from build123d import *

# Parameters (mm, degrees)
SKETCH1_W           = 25
SKETCH1_H           = 34
BOSS_EXTRUDE1_DEPTH = 5
SKETCH2_W           = 10
SKETCH2_H           = 34
BOSS_EXTRUDE2_DEPTH = 51
SKETCH3_R           = 2.8
CUT_EXTRUDE1_DEPTH  = 41
CHAMFER1_SIZE       = 4
FILLET1_R           = 4
FILLET2_R           = 4
SKETCH4_R           = 0.85
CUT_EXTRUDE2_DEPTH  = 41
SKETCH5_W           = 10
SKETCH5_H           = 20
BOSS_EXTRUDE3_DEPTH = 6
CHAMFER3_SIZE       = 15
FILLET4_R           = 10
SKETCH7_R           = 0.9
SKETCH7_R_2         = 0.85
CUT_EXTRUDE3_DEPTH  = 13


with BuildPart() as part:
    # Sketch1 → Boss-Extrude1 (new body)
    with BuildSketch(Plane(origin=(0, 0, 0), x_dir=(1, 0, 0), z_dir=(0, 1, 0))):
        Rectangle(SKETCH1_W, SKETCH1_H)
    extrude(amount=BOSS_EXTRUDE1_DEPTH)

    # Sketch2 → Boss-Extrude2 (add)
    with BuildSketch(Plane(origin=(0, 5, 0), x_dir=(1, 0, 0), z_dir=(0, 1, 0))):
        Rectangle(SKETCH2_W, SKETCH2_H)
    extrude(amount=BOSS_EXTRUDE2_DEPTH)

    # Sketch3 → Cut-Extrude1 (cut)
    with BuildSketch(Plane.ZY.offset(5)):
        with Locations((0, 46)):
            Circle(SKETCH3_R)
    extrude(amount=-CUT_EXTRUDE1_DEPTH, mode=Mode.SUBTRACT)

    # Chamfer1
    chamfer1_edges = [part.edges().sort_by_distance(p)[0] for p in [
        (-12.5, 5, 0),
        (12.5, 5, 0),
    ]]
    chamfer(chamfer1_edges, length=CHAMFER1_SIZE)

    # Fillet1
    # the kernel refuses this fillet: 4 mm, written as the material it adds along each edge
    with BuildSketch(Plane(origin=(5, 5, 17), x_dir=(1, 0, 0), z_dir=(0, 0, -1)), Plane(origin=(-5, 5, -17), x_dir=(-1, 0, 0), z_dir=(0, 0, 1))) as fillet1_piece_1:
        with BuildLine():
            CenterArc((4, -3.968626967), FILLET1_R, 97.180755781, 82.819244219)
            Line((0, -3.968626967), (-0.08, -3.968626967))
            Line((-0.08, -3.968626967), (-0.08, 0))
            Line((-0.08, 0), (0, 0.08))
            ThreePointArc((0, 0.08), (1.75, 0.08), (3.49, 0.079372539))
            Line((3.49, 0.079372539), (3.5, 0))
        make_face()
    extrude(amount=34)

    # Fillet2
    fillet2_edges = [part.edges().sort_by_distance(p)[0] for p in [
        (8.5, 5, 0),
        (-8.5, 5, 0),
    ]]
    fillet(fillet2_edges, radius=FILLET2_R)

    # Sketch4 → Cut-Extrude2 (cut)
    with BuildSketch(Plane.ZY.offset(5)):
        with Locations((6, 29.968626967)):
            Circle(SKETCH4_R)
        with Locations((13, 29.968626967)):
            Circle(SKETCH4_R)
        with Locations((2.5, 29.968626967)):
            Circle(SKETCH4_R)
        with Locations((9.5, 29.968626967)):
            Circle(SKETCH4_R)
    extrude(amount=-CUT_EXTRUDE2_DEPTH, mode=Mode.SUBTRACT)

    # Sketch5 → Boss-Extrude3 (add)
    with BuildSketch(Plane(origin=(0, 0, -17), x_dir=(-1, 0, 0), z_dir=(0, 0, -1))):
        with Locations((0, 46)):
            Rectangle(SKETCH5_W, SKETCH5_H)
    extrude(amount=BOSS_EXTRUDE3_DEPTH)

    # Chamfer3
    # the kernel refuses this chamfer: 15 mm, written as the material it adds along each edge
    with BuildSketch(Plane(origin=(-5, 36, -17), x_dir=(0, -0.9996219169112968, 0.02749587661058632), z_dir=(1, 0, 0))) as chamfer3_piece_1_section:
        Polygon((CHAMFER3_SIZE * 0.999621916911, CHAMFER3_SIZE * 0.0274958766106), (-CHAMFER3_SIZE * 0.0274958766106, CHAMFER3_SIZE * 0.999621916911), (0, 0), align=None)
    chamfer3_piece_1 = extrude(amount=10, mode=Mode.PRIVATE)
    chamfer3_piece_1 = split(chamfer3_piece_1, bisect_by=Plane(origin=(0, 29.791642651, -23), z_dir=(0, 0, 1)), keep=Keep.TOP, mode=Mode.PRIVATE)
    add(chamfer3_piece_1)

    # Fillet4
    fillet4_edges = [part.edges().sort_by_distance(p)[0] for p in [
        (0, 56, 17),
        (0, 56, -23),
    ]]
    fillet(fillet4_edges, radius=FILLET4_R)

    # Sketch7 → Cut-Extrude3 (cut)
    with BuildSketch(Plane(origin=(5, 0, 0), x_dir=(0, 0, -1), z_dir=(1, 0, 0))):
        with Locations((13.030614343, 27.851199121)):
            Circle(SKETCH7_R)
        with Locations((19.374768852, 30.809526953)):
            Circle(SKETCH7_R_2)
    extrude(amount=-CUT_EXTRUDE3_DEPTH, mode=Mode.SUBTRACT)


solid = part.part
Could you check a few things on this model? Use its own coordinates, in mm. A direction names the side the tool comes from. Give positions to 0.01 mm unless a question says otherwise; leave off trailing zeros. Order: outer loops, then holes, each group sorted by start corner. A loop starts at its lowest first (then second) coordinate and runs counter-clockwise, first axis right, second up. Notation, with made-up numbers: (33, -18) - (66, -18) arc R36 ccw to (66, 19) - close; hole circle Ø1 at (-31, 86.25). An arc over 180 degrees is marked (long way). Return JSON: item names as keys, results as strings. Group by question number.
Q1. Which directions (+Z, -Z, +X, -X, +Y, -Y) give clear straight access to the entire face, cutting with the end or side of a thin tool? Please do faces 5 (the face through (-5, 33, -3)), 6 (the face through (-0.07, 30.685, 2.957)).
Q2. Suppose I cut it at D-D, the plane z = 13. Please give me the cut outline in (x, y), and give its area (3 significant figures).
Q3. Suppose I cut it at B-B, the plane y = 44.5. Please give me the cut outline in (x, z), and give its area (3 significant figures).
Q4. Suppose I cut it at A-A, the plane z = 0. Please give me the cut outline in (x, y), and give its area (3 significant figures).
Q5. Will these pins go through, and if not, where does the flat tip stop? pin 1 Ø5 at (x, z) = (9.5, 2.5) entering from +Y; pin 2 Ø2.5 at (y, z) = (29.97, 2.5) entering from -X; pin 3 Ø1 at (x, y) = (2, 5.5) entering from -Z.
Q6. Suppose I cut it at C-C, the plane x = -1.5. Please give me the cut outline in (y, z), and give its area (3 significant figures).
Q7. Thinking about a two-plate mould opening in Z: for faces 1 (the face through (5, 33, -3)), 2 (the face through (0, 18, 17)), 3 (the face through (0, 8, -17)), 4 (the face through (0.07, 30.055, -19.767)), which applies, pulls with the +Z half, pulls with the -Z half, needs draft (parallel to the pull), parting line crosses it, or undercut?
Q8. Please list where these lines run through material, in increasing order: line 1 along Y through (x, z) = (-1.5, 6); line 2 along Y through (x, z) = (-2, 0); line 3 along Y through (x, z) = (-0.5, 2.5). Write a range as [from, to].
Resolved:
{
 "1": {"face 5": "+Z, -Z, -X, +Y", "face 6": "+X, -X"},
 "2": {"outline": "(-12.5, 0) - (12.5, 0) - (12.5, 1) - (9.29, 4.21) arc R4 ccw to (7.73, 5.18) arc R4 cw to (5, 8.97) - (5, 29.12) - (-5, 29.12) - (-5, 8.97) arc R4 cw to (-7.73, 5.18) arc R4 ccw to (-9.29, 4.21) - (-12.5, 1) - close; (-5, 30.82) - (5, 30.82) - (5, 54) - (-5, 54) - close", "area": "588 mm2"},
 "3": {"outline": "(-5, -23) - (5, -23) - (5, -2.36) - (-5, -2.36) - close; (-5, 2.36) - (5, 2.36) - (5, 17) - (-5, 17) - close", "area": "353 mm2"},
 "4": {"outline": "(-12.5, 0) - (12.5, 0) - (12.5, 1) - (9.29, 4.21) arc R4 ccw to (7.73, 5.18) arc R4 cw to (5, 8.97) - (5, 43.2) - (-5, 43.2) - (-5, 8.97) arc R4 cw to (-7.73, 5.18) arc R4 ccw to (-9.29, 4.21) - (-12.5, 1) - close; (-5, 48.8) - (5, 48.8) - (5, 56) - (-5, 56) - close", "area": "569 mm2"},
 "5": {"pin 1": "stops at y = 5.5", "pin 2": "stops at x = -5", "pin 3": "stops at z = -17"},
 "6": {"outline": "(0, -17) - (21, -17) - (27, -23) - (46, -23) arc R10 ccw to (56, -13) - (56, 7) arc R10 ccw to (46, 17) - (0, 17) - close; hole circle Ø1.8 at (27.85, -13.03); hole circle Ø1.7 at (29.97, 2.5); hole circle Ø1.7 at (29.97, 6); hole circle Ø1.7 at (29.97, 9.5); hole circle Ø1.7 at (29.97, 13); hole circle Ø1.7 at (30.81, -19.37); hole circle Ø5.6 at (46, 0)", "area": "2,010 mm2"},
 "7": {"face 1": "needs draft", "face 2": "pulls with the +Z half", "face 3": "pulls with the -Z half", "face 4": "undercut"},
 "8": {"line 1": "y = [0, 29.12], [30.82, 56]", "line 2": "y = [0, 43.2], [48.8, 56]", "line 3": "y = [0, 29.12], [30.82, 44.74], [47.26, 56]"}
}
